from build123d import *

# Parameters (mm, degrees)
FILLET1_R    = 0.4
RECPAT_COUNT = 2
RECPAT_ANGLE = 90


with BuildPart() as part:
    # BodySke → BaseBody (revolve)
    with BuildSketch(Plane.XY, mode=Mode.PRIVATE) as basebody_sk:
        with BuildLine():
            Line((5.4, 4), (5.4, 7))
            Line((5.4, 7), (2.956076559, 6.786184404))
            ThreePointArc((2.956076559, 6.786184404), (1.52557938, 6.199578276), (0.681056287, 4.904506975))
            ThreePointArc((0.681056287, 4.904506975), (0.171077054, 2.475784034), (0, 0))
            Line((0, 0), (55.4, 0))
            Line((55.4, 0), (55.4, 4))
            Line((55.4, 4), (5.4, 4))
        make_face()
    revolve(basebody_sk.sketch.rotate(Axis((0, 0, 0), (1, 0, 0)), 90), axis=Axis((0, 0, 0), (1, 0, 0)))

    # Fillet1
    fillet1_edges = [part.edges().sort_by_distance(p)[0] for p in [
        (5.4, 0, -4),
    ]]
    fillet(fillet1_edges, radius=FILLET1_R)

    # RecSkeTop → Recess section 0
    with BuildSketch(Plane(origin=(0, 0, 0), x_dir=(0, 0, -1), z_dir=(1, 0, 0))):
        with BuildLine():
            Line((-1.155, 5.25), (1.155, 5.25))
            Line((1.155, 5.25), (1.155, -5.25))
            Line((1.155, -5.25), (-1.155, -5.25))
            Line((-1.155, -5.25), (-1.155, 5.25))
        make_face()
    # RecSkeBot → Recess section 1
    with BuildSketch(Plane(origin=(4.36, 0, 0), x_dir=(0, 0, -1), z_dir=(1, 0, 0))):
        with BuildLine():
            Line((-1.155, 3.076184552), (1.155, 3.076184552))
            Line((1.155, 3.076184552), (1.155, -3.076184552))
            Line((1.155, -3.076184552), (-1.155, -3.076184552))
            Line((-1.155, -3.076184552), (-1.155, 3.076184552))
        make_face()
    recess = loft(mode=Mode.SUBTRACT)

    # RecPat: Recess ×2 about axis
    recpat_axis = Axis((0, 0, 0), (1, 0, 0))
    for i in range(1, RECPAT_COUNT):
        add(recess.rotate(recpat_axis, i * RECPAT_ANGLE / (RECPAT_COUNT - 1)), mode=Mode.SUBTRACT)

    # RecCorSke → RecessCore (revolve, cut)
    with BuildSketch(Plane.XY, mode=Mode.PRIVATE) as recesscore_sk:
        Polygon((0, 0), (0, 2.541), (4.36, 2.2361191), (5.086559139, 0), align=None)
    revolve(recesscore_sk.sketch.rotate(Axis((0, 0, 0), (1, 0, 0)), 90), axis=Axis((0, 0, 0), (1, 0, 0)), mode=Mode.SUBTRACT)


solid = part.part
Work out the finished part from the listing and answer in its coordinate system (mm). A direction names the side the tool comes from. Give positions to 0.01 mm unless a question says otherwise; leave off trailing zeros. Write each loop counter-clockwise with the first axis right and the second up, starting at its lowest first coordinate (ties: lowest second). Pieces come first, ordered by that corner, then holes.
Q1. For a pull along Z with two mould halves and no side action, classify faces 4 (the face through (3.618, -2.056, 6.528)), 5 (the face through (2.299, -1.676, 1.69)), 6 (the face through (5.4, 5, 0)), 7 (the face through (2.299, 1.69, 1.676)) as released by +Z, released by -Z, zero draft, split by the parting line, or undercut.
Answer:
face 4: split by the parting line
face 5: undercut
face 6: zero draft
face 7: undercut
Q2. A tool of negligible diameter and unlimited length cuts with its end or side. For faces 1 (the face through (2.55, 0.02, -3.98)), 2 (the face through (55.4, 0, 0)), 3 (the face through (30.253, 3.905, -0.867)), from which of +Z, -Z, +X, -X, +Y, -Y can it reach the whole face along a straight path? Write none if from no direction.
Answer:
face 1: -X
face 2: +Z, -Z, +X, +Y, -Y
face 3: +X
Q3. Straight lines are drawn through the part: L1, parallel to X at y = -1, z = -2.25; L2, parallel to Y at x = 15, z = 0; L3, parallel to X at y = -1.25, z = -6. For each, find the intervals that lie inside material, in ascending order.
Answer:
L1: x = 4.36 to 55.4
L2: y = -4 to 4
L3: x = 1.44 to 5.4
Q4. The part is cut by section A-A on x = 22. Give the vertices of the cut face in (y, z), and give its area (3 significant figures).
Answer:
outline: circle Ø8 at (0, 0)
area: 50.3 mm2
Q5. Given pin 1 (0.9 mm diameter, centred on y = 0.5, z = 2.5, fed in from -X); pin 2 (6 mm diameter, centred on x = 29, y = 3, fed in from +Z); pin 3 (3 mm diameter, centred on x = 23, z = 3.5, fed in from -Y), each flat-ended and moving along its own axis, determine where each tip first touches the part or whether it passes through.
Answer:
pin 1: stops at x = 4.36
pin 2: stops at z = 4
pin 3: stops at y = -3.46
